Verification items for the finished model (mm, model axes). A direction names the side the tool comes from. Give positions to 0.01 mm unless a question says otherwise; leave off trailing zeros. Loops run counter-clockwise (first coordinate to the right, second up) from the corner with the lowest first, then second, coordinate; pieces in that order, holes last. Notation, with made-up numbers: (89.5, 20.25) - (136.5, 20.25) arc R28 ccw to (136.5, 59.25) - close; hole circle Ø5 at (83, 36.5). An arc over 180 degrees is marked (long way). Answer in a Markdown table with one row per item.
```python
from build123d import *

# Parameters (mm, degrees)
SKETCH1_W           = 40
SKETCH1_H           = 7
BOSS_EXTRUDE3_DEPTH = 120
CUT_EXTRUDE3_DEPTH  = 120
CUT_EXTRUDE4_DEPTH  = 120
BOSS_EXTRUDE4_DEPTH = 120
BOSS_EXTRUDE5_DEPTH = 120


with BuildPart() as part:
    # Sketch1 → Boss-Extrude3 (new body)
    with BuildSketch(Plane(origin=(0, 0, 0), x_dir=(1, 0, 0), z_dir=(0, 1, 0))):
        with Locations((-32.467727981, -13.5274909)):
            Rectangle(SKETCH1_W, SKETCH1_H)
    extrude(amount=BOSS_EXTRUDE3_DEPTH)

    # Sketch6 → Cut-Extrude3 (cut)
    with BuildSketch(Plane(origin=(0, 120, 0), x_dir=(1, 0, 0), z_dir=(0, 1, 0))):
        Polygon((-52.467727981, -17.0274909), (-52.467727981, -10.0274909), (-45.467727981, -17.0274909), align=None)
    extrude(amount=-CUT_EXTRUDE3_DEPTH, mode=Mode.SUBTRACT)

    # Sketch7 → Cut-Extrude4 (cut)
    with BuildSketch(Plane(origin=(0, 120, 0), x_dir=(1, 0, 0), z_dir=(0, 1, 0))):
        Polygon((-12.467727981, -17.0274909), (-12.467727981, -10.0274909), (-19.467727981, -17.0274909), align=None)
    extrude(amount=-CUT_EXTRUDE4_DEPTH, mode=Mode.SUBTRACT)

    # Sketch8 → Boss-Extrude4 (add)
    with BuildSketch(Plane(origin=(0, 120, 0), x_dir=(1, 0, 0), z_dir=(0, 1, 0))):
        Polygon((-49.816077551, -12.679141329), (-52.11417459, -14.977238368), (-53.351611457, -13.739801501), (-54.942601715, -15.330791759), (-50.699961028, -19.573432446), (-49.10897077, -17.982442188), (-50.346407637, -16.745005321), (-48.048310598, -14.446908282), align=None)
    extrude(amount=-BOSS_EXTRUDE4_DEPTH)

    # Sketch9 → Boss-Extrude5 (add)
    with BuildSketch(Plane(origin=(0, 120, 0), x_dir=(1, 0, 0), z_dir=(0, 1, 0))):
        Polygon((-17.172372993, -14.732135912), (-14.874275954, -17.030232951), (-16.111712821, -18.267669818), (-14.520722564, -19.858660076), (-10.278081876, -15.616019388), (-11.869072134, -14.025029131), (-13.106509001, -15.262465998), (-15.40460604, -12.964368959), align=None)
    extrude(amount=-BOSS_EXTRUDE5_DEPTH)


solid = part.part
```
Q1. Go/stop test with flat-tipped pins: P1, Ø1.5, axis at y = 23.5, z = 12, coming from the -X side; P2, Ø4, axis at y = 26.5, z = 15.5, coming from the -X side; P3, Ø13, axis at x = -36, y = 30.5, coming from the +Z side. Record where each tip stops, or that it passes through.
Completed:
| item | result |
|---|---|
| P1 | x = -51.25 |
| P2 | x = -54.94 |
| P3 | z = 17.03 |
Q2. Tool access check on faces 1 (the face through (-46.776, 60.84, 15.719)), 2 (the face through (-13.92, 60.84, 11.48)), 3 (the face through (-16.039, 60.84, 15.865)), 4 (the face through (-51.16, 60.84, 11.335)). Record the directions out of +Z, -Z, +X, -X, +Y, -Y that give a thin tool (end or side, any length) a straight path to the whole face; none if there is none.
Completed:
| item | result |
|---|---|
| face 1 | +Z, +Y, -Y |
| face 2 | +X, +Y, -Y |
| face 3 | +Y, -Y |
| face 4 | -X, +Y, -Y |
Q3. Sectioned sample at B-B (x = -38.5). Record the cut outline in (y, z).
Completed:
| item | result |
|---|---|
| outline | (0, 10.03) - (120, 10.03) - (120, 17.03) - (0, 17.03) - close |
Q4. Sectioned sample at C-C (z = 11.5). Record the cut outline in (x, y), and give its area (3 significant figures).
Completed:
| item | result |
|---|---|
| outline | (-51, 0) - (-13.94, 0) - (-13.94, 120) - (-51, 120) - close |
| area | 4,450 mm^2 |
Q5. Thickness scan on line 1 (X direction, y = 55, z = 16); line 2 (X direction, y = 74, z = 15.5); line 3 (Z direction, x = -13, y = 105). Record the ranges inside material, lowest first.
Completed:
| item | result |
|---|---|
| line 1 | -54.27 to -49.6, -46.5 to -18.44, -15.9 to -10.66 |
| line 2 | -54.77 to -49.1, -47 to -17.94, -16.4 to -10.39 |
| line 3 | 10.03 to 10.56, 15.16 to 18.34 |
Q6. Sectioned sample at A-A (y = 22.5). Record the cut outline in (x, z) (1 decimal), and give its area (3 significant figures).
Completed:
| item | result |
|---|---|
| outline | (-54.9, 15.3) - (-53.4, 13.7) - (-52.1, 15) - (-49.8, 12.7) - (-52.5, 10) - (-12.5, 10) - (-15.4, 13) - (-13.1, 15.3) - (-11.9, 14) - (-10.3, 15.6) - (-14.5, 19.9) - (-16.1, 18.3) - (-14.9, 17) - (-17.2, 14.7) - (-19.5, 17) - (-45.5, 17) - (-48, 14.4) - (-50.3, 16.7) - (-49.1, 18) - (-50.7, 19.6) - close |
| area | 274 mm^2 |
